Design review of the part built by this model. Coordinates are the model's own, in mm. A direction names the side the tool comes from. Round coordinates to 2 decimals unless told otherwise and drop trailing zeros. Write each loop counter-clockwise with the first axis right and the second up, starting at its lowest first coordinate (ties: lowest second). Pieces come first, ordered by that corner, then holes. Notation, with made-up numbers: (80.25, -36) - (138.25, -36) arc R19 ccw to (138.25, -25) - close; hole circle Ø2 at (38.25, 0). An arc over 180 degrees is marked (long way). Use one line per item in the form item = value.
```python
from build123d import *

# Parameters (mm, degrees)
SKETCH1_R           = 13.9
SKETCH1_R_2         = 1.4
BOSS_EXTRUDE1_DEPTH = 5


with BuildPart() as part:
    # Sketch1 → Boss-Extrude1 (new body)
    with BuildSketch(Plane(origin=(0, 0, 0), x_dir=(1, 0, 0), z_dir=(0, 1, 0))):
        with BuildLine():
            Line((26.464466094, -43.035533906), (33.964466094, -35.535533906))
            ThreePointArc((33.964466094, -35.535533906), (37.5, -34.071067812), (41.035533906, -35.535533906))
            Line((41.035533906, -35.535533906), (48.535533906, -43.035533906))
            ThreePointArc((48.535533906, -43.035533906), (50.15765065, -44.119397663), (52.071067812, -44.5))
            Line((52.071067812, -44.5), (81, -44.5))
            ThreePointArc((81, -44.5), (88.071067812, -41.571067812), (91, -34.5))
            Line((91, -34.5), (91, 34.5))
            ThreePointArc((91, 34.5), (88.071067812, 41.571067812), (81, 44.5))
            Line((81, 44.5), (52.071067812, 44.5))
            ThreePointArc((52.071067812, 44.5), (50.15765065, 44.119397663), (48.535533906, 43.035533906))
            Line((48.535533906, 43.035533906), (41.035533906, 35.535533906))
            ThreePointArc((41.035533906, 35.535533906), (37.5, 34.071067812), (33.964466094, 35.535533906))
            Line((33.964466094, 35.535533906), (26.464466094, 43.035533906))
            ThreePointArc((26.464466094, 43.035533906), (24.84234935, 44.119397663), (22.928932188, 44.5))
            Line((22.928932188, 44.5), (-81, 44.5))
            ThreePointArc((-81, 44.5), (-88.071067812, 41.571067812), (-91, 34.5))
            Line((-91, 34.5), (-91, -34.5))
            ThreePointArc((-91, -34.5), (-88.071067812, -41.571067812), (-81, -44.5))
            Line((-81, -44.5), (22.928932188, -44.5))
            ThreePointArc((22.928932188, -44.5), (24.84234935, -44.119397663), (26.464466094, -43.035533906))
        make_face()
        with Locations((-8, 0)):
            Circle(SKETCH1_R, mode=Mode.SUBTRACT)
        with Locations((-30.273863607, 8.131727984)):
            Circle(SKETCH1_R_2, mode=Mode.SUBTRACT)
        with Locations((-16.131727984, 22.273863607)):
            Circle(SKETCH1_R_2, mode=Mode.SUBTRACT)
        with Locations((0.131727984, 22.273863607)):
            Circle(SKETCH1_R_2, mode=Mode.SUBTRACT)
        with Locations((14.273863607, 8.131727984)):
            Circle(SKETCH1_R_2, mode=Mode.SUBTRACT)
        with Locations((14.273863607, -8.131727984)):
            Circle(SKETCH1_R_2, mode=Mode.SUBTRACT)
        with Locations((0.131727984, -22.273863607)):
            Circle(SKETCH1_R_2, mode=Mode.SUBTRACT)
        with Locations((-16.131727984, -22.273863607)):
            Circle(SKETCH1_R_2, mode=Mode.SUBTRACT)
        with Locations((-30.273863607, -8.131727984)):
            Circle(SKETCH1_R_2, mode=Mode.SUBTRACT)
        with Locations((-75, -37.5)):
            Circle(SKETCH1_R_2, mode=Mode.SUBTRACT)
        with Locations((-57, -39.5)):
            Circle(SKETCH1_R_2, mode=Mode.SUBTRACT)
        with Locations((-18, -39.5)):
            Circle(SKETCH1_R_2, mode=Mode.SUBTRACT)
        with Locations((0, -37.5)):
            Circle(SKETCH1_R_2, mode=Mode.SUBTRACT)
        with Locations((18, -39.5)):
            Circle(SKETCH1_R_2, mode=Mode.SUBTRACT)
        with Locations((57, -39.5)):
            Circle(SKETCH1_R_2, mode=Mode.SUBTRACT)
        with Locations((75, -37.5)):
            Circle(SKETCH1_R_2, mode=Mode.SUBTRACT)
        with Locations((86, -18)):
            Circle(SKETCH1_R_2, mode=Mode.SUBTRACT)
        with Locations((86, 18)):
            Circle(SKETCH1_R_2, mode=Mode.SUBTRACT)
        with Locations((75, 37.5)):
            Circle(SKETCH1_R_2, mode=Mode.SUBTRACT)
        with Locations((57, 39.5)):
            Circle(SKETCH1_R_2, mode=Mode.SUBTRACT)
        with Locations((18, 39.5)):
            Circle(SKETCH1_R_2, mode=Mode.SUBTRACT)
        with Locations((0, 37.5)):
            Circle(SKETCH1_R_2, mode=Mode.SUBTRACT)
        with Locations((-18, 39.5)):
            Circle(SKETCH1_R_2, mode=Mode.SUBTRACT)
        with Locations((-57, 39.5)):
            Circle(SKETCH1_R_2, mode=Mode.SUBTRACT)
        with Locations((-75, 37.5)):
            Circle(SKETCH1_R_2, mode=Mode.SUBTRACT)
        with Locations((-86, 18)):
            Circle(SKETCH1_R_2, mode=Mode.SUBTRACT)
        with Locations((-86, -18)):
            Circle(SKETCH1_R_2, mode=Mode.SUBTRACT)
    extrude(amount=BOSS_EXTRUDE1_DEPTH)


solid = part.part
```
Q1. To check wall thickness, follow line 1 along Z through (x, y) = (-75, 2.85); line 2 along X through (y, z) = (2.95, 18); line 3 along Z through (x, y) = (57, 3.65). State the ranges of each line that lie inside material, in increasing order. Write a range as from..to.
Calculated:
line_1 = -44.5..-38.9, -36.1..36.1, 38.9..44.5
line_2 = -91..-87.4, -84.6..84.6, 87.4..91
line_3 = -44.5..-40.9, -38.1..38.1, 40.9..44.5
Q2. Machinability: for faces 1 (the cylindrical face through (24.82, 2.46, 44.13)), 2 (the cylindrical face through (24.87, 2.46, -44.11)), 3 (the cylindrical face through (4.84, 2.46, 5.32)), which of the approach directions +Z, -Z, +X, -X, +Y, -Y give a long, thin tool a straight path to every point of the face, cutting with its end or side? Answer none if there is none.
Calculated:
face_1 = +Z, +Y, -Y
face_2 = -Z, +Y, -Y
face_3 = +Y, -Y
Q3. For P1, Ø2, axis at x = -30.27, z = 8.13, coming from the -Y side, flat-tipped, find the tip position at first contact; note if it passes through.
Calculated:
P1 = through
Q4. We need section A-A on x = -9.5. Write out the cut boundary in (y, z), then the cut area to 3 significant figures.
Calculated:
outline = (0, -44.5) - (5, -44.5) - (5, -13.82) - (0, -13.82) - close; (0, 13.82) - (5, 13.82) - (5, 44.5) - (0, 44.5) - close
area = 307 mm2
Q5. We need section B-B on y = 3.85. State how many separate pieces and enclosed holes the cut face has, then the cut area to 3 significant figures.
Calculated:
separate_pieces = 1
enclosed_holes = 27
area = 15,000 mm2
Q6. Draft analysis for pull direction X (two halves, no side actions). For faces 4 (the cylindrical face through (87.99, 2.46, 41.65)), 5 (the cylindrical face through (37.55, 2.46, -34.07)), 6 (the cylindrical face through (-87.99, 2.46, -41.65)), state which applies: released by +X, released by -X, zero draft, split by the parting line, or undercut.
Calculated:
face_4 = released by +X
face_5 = undercut
face_6 = released by -X
